from build123d import *

# Parameters (mm, degrees)
BOSS_EXTRUDE1_DEPTH     = 3.81
SKETCH3_W               = 41.91
SKETCH3_H               = 2.286
BOSS_EXTRUDE2_DEPTH     = 3.048
SKETCH4_W               = 41.91
SKETCH4_H               = 1.3716
BOSS_EXTRUDE3_DEPTH     = 2.54
CUT_EXTRUDE1_DEPTH      = 54.324878809
CUT_EXTRUDE1_DEPTH_BACK = 54.324878809
SKETCH5_R               = 1.27


with BuildPart() as part:
    # Sketch2 → Boss-Extrude1 (new body)
    with BuildSketch(Plane(origin=(0, 0, -1.651), x_dir=(-1, 0, 0), z_dir=(0, 0, -1))):
        with BuildLine():
            Line((-44.45, 26.67), (-44.45, 5.378493099))
            Line((-44.45, 5.378493099), (-44.45, 2.54))
            ThreePointArc((-44.45, 2.54), (-43.706051224, 0.743948776), (-41.91, 0))
            Line((-41.91, 0), (-6.35, 0))
            ThreePointArc((-6.35, 0), (-4.553948776, -0.743948776), (-3.81, -2.54))
            Line((-3.81, -2.54), (-3.81, -22.86))
            Line((-3.81, -22.86), (-3.81, -25.4))
            Line((-3.81, -25.4), (38.1, -25.4))
            Line((38.1, -25.4), (38.1, -22.86))
            Line((38.1, -22.86), (38.1, -16.8275))
            Line((38.1, -16.8275), (30.48, -16.8275))
            ThreePointArc((30.48, -16.8275), (28.683948776, -17.571448776), (27.94, -19.3675))
            Line((27.94, -19.3675), (27.94, -19.812))
            Line((27.94, -19.812), (3.81, -19.812))
            Line((3.81, -19.812), (3.81, -1.778))
            ThreePointArc((3.81, -1.778), (4.553948776, 0.018051224), (6.35, 0.762))
            Line((6.35, 0.762), (29.21, 0.762))
            ThreePointArc((29.21, 0.762), (31.006051224, 0.018051224), (31.75, -1.778))
            Line((31.75, -1.778), (31.75, -5.2705))
            ThreePointArc((31.75, -5.2705), (32.493948776, -7.066551224), (34.29, -7.8105))
            Line((34.29, -7.8105), (41.91, -7.8105))
            ThreePointArc((41.91, -7.8105), (43.706051224, -7.066551224), (44.45, -5.2705))
            Line((44.45, -5.2705), (44.45, 26.67))
            ThreePointArc((44.45, 26.67), (43.706051224, 28.466051224), (41.91, 29.21))
            Line((41.91, 29.21), (-41.91, 29.21))
            ThreePointArc((-41.91, 29.21), (-43.706051224, 28.466051224), (-44.45, 26.67))
        make_face()
    extrude(amount=BOSS_EXTRUDE1_DEPTH)

    # Sketch3 → Boss-Extrude2 (add)
    with BuildSketch(Plane.XY.offset(-1.651)):
        with Locations((-17.145, -24.257)):
            Rectangle(SKETCH3_W, SKETCH3_H)
    extrude(amount=BOSS_EXTRUDE2_DEPTH)

    # Sketch4 → Boss-Extrude3 (add)
    with BuildSketch(Plane(origin=(0, -23.114, 0), x_dir=(1, 0, 0), z_dir=(0, 1, 0))):
        with Locations((-17.145, -0.7112)):
            Rectangle(SKETCH4_W, SKETCH4_H)
    extrude(amount=BOSS_EXTRUDE3_DEPTH)

    # Sketch5 → Cut-Extrude1 (cut, two sides: drawn at the far end of the back side and taken through both)
    with BuildSketch(Plane.XY.offset(-1.651).offset(-CUT_EXTRUDE1_DEPTH_BACK)):
        with Locations((-34.29, 19.05)):
            Circle(SKETCH5_R)
        with Locations((34.29, 19.05)):
            Circle(SKETCH5_R)
        with Locations((-34.29, -19.05)):
            Circle(SKETCH5_R)
    extrude(amount=CUT_EXTRUDE1_DEPTH + CUT_EXTRUDE1_DEPTH_BACK, mode=Mode.SUBTRACT)


solid = part.part
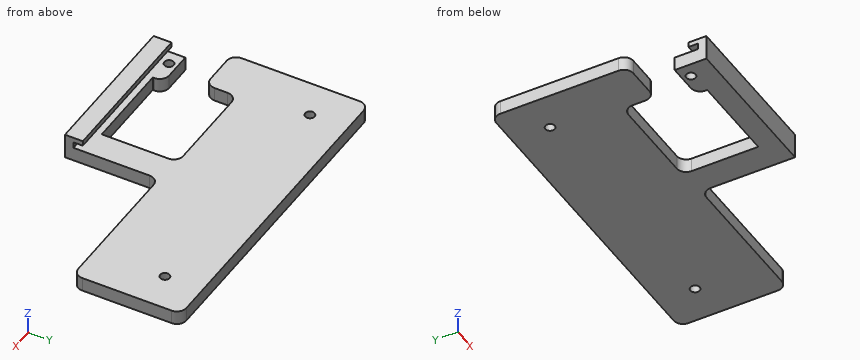
Source: CAD feature listing. Evaluate the final solid. Frame: model axes, mm. Coordinates: 2 decimals unless noted, no trailing zeros. Loops run counter-clockwise (first coordinate to the right, second up) from the corner with the lowest first, then second, coordinate; pieces in that order, holes last. Notation, with made-up numbers: (75.25, 42) -> (109.25, 42) arc R30 ccw to (109.25, 69) -> close; hole circle Ø5 at (43.5, 29.5). An arc over 180 degrees is marked (long way). Answer in a Markdown table with one row per item. Add a question column.
Q1. Ray query, line 1 along Y through (x, z) = (-34.29, -2.8); line 2 along X through (y, z) = (19.05, -3.6); line 3 along X through (y, z) = (-19.05, -3.3). Return the intervals inside material, ascending.
Q2. Contact query for flat-ended pins moving along their axis: pin 1 Ø4 at (y, z) = (-19, -3) entering from -X; pin 2 Ø4 at (y, z) = (-3, -2.5) entering from +X; pin 3 Ø3 at (x, y) = (-4.5, -18.5) entering from +Z; pin 4 Ø1.5 at (x, y) = (34.29, 19.05) entering from -Z. Output: stop coordinate, or through.
Q3. Section B-B on x = 34.29. Return the cut outline in (y, z).
Q4. Section A-A on y = 19.05. Return the cut outline in (x, z).
Q5. Section C-C on z = -2.5. Return the cut outline in (x, y).
Q6. Section D-D on x = -13. Return the cut outline in (y, z), and give its area (3 significant figures).
Computed values:
| question | item | result |
|---|---|---|
| 1 | line 1 | y = -25.4 to -20.32, -17.78 to -16.83, -7.81 to 17.78, 20.32 to 29.21 |
| 1 | line 2 | x = -44.45 to -35.56, -33.02 to 33.02, 35.56 to 44.45 |
| 1 | line 3 | x = -38.1 to -35.56, -33.02 to -27.96, -3.81 to 3.81 |
| 2 | pin 1 | stops at x = -38.1 |
| 2 | pin 2 | stops at x = 4.33 |
| 2 | pin 3 | stops at z = -1.65 |
| 2 | pin 4 | passes through |
| 3 | outline | (0, -5.46) -> (17.78, -5.46) -> (17.78, -1.65) -> (0, -1.65) -> close; (20.32, -5.46) -> (29.21, -5.46) -> (29.21, -1.65) -> (20.32, -1.65) -> close |
| 4 | outline | (-44.45, -5.46) -> (-35.56, -5.46) -> (-35.56, -1.65) -> (-44.45, -1.65) -> close; (-33.02, -5.46) -> (33.02, -5.46) -> (33.02, -1.65) -> (-33.02, -1.65) -> close; (35.56, -5.46) -> (44.45, -5.46) -> (44.45, -1.65) -> (35.56, -1.65) -> close |
| 5 | outline | (-44.45, -5.27) arc R2.54 ccw to (-41.91, -7.81) -> (-34.29, -7.81) arc R2.54 ccw to (-31.75, -5.27) -> (-31.75, -1.78) arc R2.54 cw to (-29.21, 0.76) -> (-6.35, 0.76) arc R2.54 cw to (-3.81, -1.78) -> (-3.81, -19.81) -> (-27.94, -19.81) -> (-27.94, -19.37) arc R2.54 ccw to (-30.48, -16.83) -> (-38.1, -16.83) -> (-38.1, -25.4) -> (3.81, -25.4) -> (3.81, -2.54) arc R2.54 cw to (6.35, 0) -> (41.91, 0) arc R2.54 ccw to (44.45, 2.54) -> (44.45, 26.67) arc R2.54 ccw to (41.91, 29.21) -> (-41.91, 29.21) arc R2.54 ccw to (-44.45, 26.67) -> close; hole circle Ø2.54 at (-34.29, -19.05); hole circle Ø2.54 at (-34.29, 19.05); hole circle Ø2.54 at (34.29, 19.05) |
| 6 | outline | (-25.4, -5.46) -> (-19.81, -5.46) -> (-19.81, -1.65) -> (-23.11, -1.65) -> (-23.11, 0.03) -> (-20.57, 0.03) -> (-20.57, 1.4) -> (-25.4, 1.4) -> close; (0.76, -5.46) -> (29.21, -5.46) -> (29.21, -1.65) -> (0.76, -1.65) -> close |
| 6 | area | 140 mm^2 |
